```python
from build123d import *

# Parameters (mm, degrees)
SKETCH2_R           = 1.25
SKETCH2_W           = 6.35
SKETCH2_H           = 6.5
BOSS_EXTRUDE1_DEPTH = 1
BOSS_EXTRUDE2_START = -2.032
SKETCH2_3_R         = 1.25
BOSS_EXTRUDE2_DEPTH = 2.032


with BuildPart() as part:
    # Sketch2 → Boss-Extrude1 (new body)
    # profile 1 of 3: a face of its own
    with BuildSketch(Plane(origin=(0, 0, 0), x_dir=(1, 0, 0), z_dir=(0, 1, 0))):
        with BuildLine():
            Line((-3.175, 3.25), (-6.425, 3.25))
            ThreePointArc((-6.425, 3.25), (-9.675, 0), (-6.425, -3.25))
            Line((-6.425, -3.25), (-3.175, -3.25))
            Line((-3.175, -3.25), (-3.175, 3.25))
        make_face()
        with Locations(Location((-6.425, 0, 0), (0, 0, 270))):
            Circle(SKETCH2_R, mode=Mode.SUBTRACT)
    # profile 2 of 3: a face of its own
    with BuildSketch(Plane(origin=(0, 0, 0), x_dir=(1, 0, 0), z_dir=(0, 1, 0))):
        Rectangle(SKETCH2_W, SKETCH2_H)
    # profile 3 of 3: a face of its own
    with BuildSketch(Plane(origin=(0, 0, 0), x_dir=(1, 0, 0), z_dir=(0, 1, 0))):
        with BuildLine():
            Line((6.425, 3.25), (3.175, 3.25))
            Line((3.175, 3.25), (3.175, -3.25))
            Line((3.175, -3.25), (6.425, -3.25))
            ThreePointArc((6.425, -3.25), (9.675, 0), (6.425, 3.25))
        make_face()
        with Locations(Location((6.425, 0, 0), (0, 0, 270))):
            Circle(SKETCH2_R, mode=Mode.SUBTRACT)
    extrude(amount=BOSS_EXTRUDE1_DEPTH)

    # Sketch2_3 → Boss-Extrude2 (add)
    # profile 1 of 2: a face of its own
    with BuildSketch(Plane(origin=(0, 0, 0), x_dir=(1, 0, 0), z_dir=(0, 1, 0)).offset(BOSS_EXTRUDE2_START)):
        with BuildLine():
            Line((-3.175, 3.25), (-6.425, 3.25))
            ThreePointArc((-6.425, 3.25), (-9.675, 0), (-6.425, -3.25))
            Line((-6.425, -3.25), (-3.175, -3.25))
            Line((-3.175, -3.25), (-3.175, 3.25))
        make_face()
        with Locations(Location((-6.425, 0, 0), (0, 0, 270))):
            Circle(SKETCH2_3_R, mode=Mode.SUBTRACT)
    # profile 2 of 2: a face of its own
    with BuildSketch(Plane(origin=(0, 0, 0), x_dir=(1, 0, 0), z_dir=(0, 1, 0)).offset(BOSS_EXTRUDE2_START)):
        with BuildLine():
            Line((6.425, 3.25), (3.175, 3.25))
            Line((3.175, 3.25), (3.175, -3.25))
            Line((3.175, -3.25), (6.425, -3.25))
            ThreePointArc((6.425, -3.25), (9.675, 0), (6.425, 3.25))
        make_face()
        with Locations(Location((6.425, 0, 0), (0, 0, 270))):
            Circle(SKETCH2_3_R, mode=Mode.SUBTRACT)
    extrude(amount=BOSS_EXTRUDE2_DEPTH)


solid = part.part
```
Part model, mm, in its own coordinate system. A direction names the side the tool comes from. Give positions to 0.01 mm unless a question says otherwise; leave off trailing zeros. Write each loop counter-clockwise with the first axis right and the second up, starting at its lowest first coordinate (ties: lowest second). Pieces come first, ordered by that corner, then holes. Notation, with made-up numbers: (69, -17.75) -> (111, -17.75) arc R19 cw to (111, -9.75) -> close; hole circle Ø11 at (13.25, -37). An arc over 180 degrees is marked (long way). Put each result on its own line as item: value. Start each with the question number.
Item 1: Cut at A-A (y = -1.1). List the corners of the cut face in (x, z) (3 decimals).
Item 2: Wall check: L1, parallel to X at y = -1.4, z = 0 (3 decimals); L2, parallel to X at y = 0.35, z = 0 (3 decimals); L3, parallel to X at y = -0.3, z = 0.5 (3 decimals). Give the ranges that are in metal, low to high. Write a range as [from, to].
Item 3: Pin check, flat tips, straight feed: pin 1 Ø0.6 at (y, z) = (-1, -0.5) entering from +X; pin 2 Ø3 at (x, z) = (1, -1) entering from -Y; pin 3 Ø2 at (x, z) = (6.425, 0) entering from -Y; pin 4 Ø1 at (y, z) = (0.5, 1) entering from -X. Stop position of each tip, or through.
Item 4: Cut at D-D (x = 5.5). List the corners of the cut face in (y, z).
Item 5: Cut at C-C (y = 0.55). List the corners of the cut face in (x, z) (3 decimals).
Item 6: Pull direction X, two halves, no side cores. Call faces 3 (the face through (0, 0, 0)), 4 (the face through (0.1, 0.5, -3.25)), 5 (the face through (-9.674, -0.537, -0.071)): pulls with the +X half, pulls with the -X half, needs draft (parallel to the pull), parting line crosses it, or undercut.
Item 7: Cut at B-B (z = 0). List the corners of the cut face in (x, y) (3 decimals).
Item 8: Which spindle directions (+Z, -Z, +X, -X, +Y, -Y) get a long thin tool onto all of the face, cutting with end or side? Do faces 1 (the face through (-0.1, 0.5, 3.25)), 2 (the face through (3.175, -1, 0)). Say none if no direction does.
Answer list:
1. outline: (-6.425, -3.25) -> (-3.175, -3.25) -> (-3.175, 3.25) -> (-6.425, 3.25) arc R3.25 ccw to start; (3.175, -3.25) -> (6.425, -3.25) arc R3.25 ccw to (6.425, 3.25) -> (3.175, 3.25) -> close; hole circle Ø2.5 at (-6.425, 0); hole circle Ø2.5 at (6.425, 0)
2. L1: x = [-9.675, -7.675], [-5.175, -3.175], [3.175, 5.175], [7.675, 9.675]
2. L2: x = [-9.675, -7.675], [-5.175, 5.175], [7.675, 9.675]
2. L3: x = [-9.636, -7.571], [-5.279, -3.175], [3.175, 5.279], [7.571, 9.636]
3. pin 1: stops at x = 9.67
3. pin 2: stops at y = 0
3. pin 3: passes through
3. pin 4: stops at x = -9.64
4. outline: (-2.03, -3.25) -> (1, -3.25) -> (1, -0.84) -> (-2.03, -0.84) -> close; (-2.03, 0.84) -> (1, 0.84) -> (1, 3.25) -> (-2.03, 3.25) -> close
5. outline: (-6.425, -3.25) -> (6.425, -3.25) arc R3.25 ccw to (6.425, 3.25) -> (-6.425, 3.25) arc R3.25 ccw to start; hole circle Ø2.5 at (-6.425, 0); hole circle Ø2.5 at (6.425, 0)
6. face 3: undercut
6. face 4: needs draft
6. face 5: pulls with the -X half
7. outline: (-9.675, -2.032) -> (-7.675, -2.032) -> (-7.675, 1) -> (-9.675, 1) -> close; (-5.175, -2.032) -> (-3.175, -2.032) -> (-3.175, 0) -> (3.175, 0) -> (3.175, -2.032) -> (5.175, -2.032) -> (5.175, 1) -> (-5.175, 1) -> close; (7.675, -2.032) -> (9.675, -2.032) -> (9.675, 1) -> (7.675, 1) -> close
8. face 1: +Z, +X, -X, +Y, -Y
8. face 2: +Z, -Z, -Y
